Work out the finished part from the listing and answer in its coordinate system (mm). A direction names the side the tool comes from. Round coordinates to 2 decimals unless told otherwise and drop trailing zeros. Order: outer loops, then holes, each group sorted by start corner. A loop starts at its lowest first (then second) coordinate and runs counter-clockwise, first axis right, second up. Notation, with made-up numbers: M 15.5,-15 L 68.5,-15 A27 ccw 68.5,14 Z; hole C 74.5,-18 d9. An arc over 180 degrees is marked long. Return JSON: item names as keys, results as strings.
from build123d import *

# Parameters (mm, degrees)
F0_R     = 44.45
F1_DEPTH = 165.1
F2_R     = 38.1
F3_DEPTH = 254
F4_W     = 86.713158
F4_H     = 16.258716
F5_DEPTH = 25.4
F6_W     = 50.8
F6_H     = 16.258716
F7_DEPTH = 25.4
F8_R     = 2.54
F9_DEPTH = 25.4


with BuildPart() as f1:
    # F0 (on Front) → F1 (new body)
    with BuildSketch(Plane.XZ):
        Circle(F0_R)
    extrude(amount=F1_DEPTH)

    # F2 (on face) → F3 (cut)
    with BuildSketch(Plane.XZ.offset(165.1)):
        Circle(F2_R)
    extrude(amount=-F3_DEPTH, mode=Mode.SUBTRACT)

    # F4 (on Front) → F5 (join)
    with BuildSketch(Plane.XZ):
        Rectangle(F4_W, F4_H)
    extrude(amount=F5_DEPTH)

    # F6 (on face) → F7 (cut)
    with BuildSketch(Plane(origin=(0, 0, 0), x_dir=(-1, 0, 0), z_dir=(0, 1, 0))):
        Rectangle(F6_W, F6_H)
    extrude(amount=-F7_DEPTH, mode=Mode.SUBTRACT)

    # F8 (on face) → F9 (join)
    with BuildSketch(Plane.XZ.offset(25.4)):
        with Locations((31.311311, 0)):
            Circle(F8_R)
        with Locations((-31.311311, 0)):
            Circle(F8_R)
    extrude(amount=F9_DEPTH)


solid = f1.part
Item 1: Find section A-A (z = 0). Determine the outline of the cut face in (x, y), plus the area to 3 significant figures.
Output:
{"outline": "M -44.45,-165.1 L -38.1,-165.1 L -38.1,-25.4 L -33.85,-25.4 L -33.85,-50.8 L -28.77,-50.8 L -28.77,-25.4 L -25.4,-25.4 L -25.4,0 L -44.45,0 Z; M 25.4,-25.4 L 28.77,-25.4 L 28.77,-50.8 L 33.85,-50.8 L 33.85,-25.4 L 38.1,-25.4 L 38.1,-165.1 L 44.45,-165.1 L 44.45,0 L 25.4,0 Z", "area": "3,000 mm^2"}
Item 2: Find section B-B (x = 0). Determine the outline of the cut face in (y, z), plus the area to 3 significant figures.
Output:
{"outline": "M -165.1,-44.45 L 0,-44.45 L 0,-38.1 L -165.1,-38.1 Z; M -165.1,38.1 L 0,38.1 L 0,44.45 L -165.1,44.45 Z", "area": "2,100 mm^2"}
Item 3: Which of the six approach directions +Z, -Z, +X, -X, +Y, -Y give full straight-line access (tool end or side, diameter ignored) to faces 1 (the flat face through (33, -165.1, 20)), 2 (the cylindrical face through (28.774, -37.922, 0.112)), 3 (the flat face through (-31, -13, -8.129))?
Output:
{"face 1": "+Z, -Z, +X, -X, -Y", "face 2": "-Y", "face 3": "+Y, -Y"}
Item 4: Each of these flat-tipped pins is pushed along its axis until it touches: pin 1 (8 mm diameter, centred on y = -128, z = 24, fed in from +X); pin 2 (6 mm diameter, centred on x = 33, y = -15.5, fed in from -Z); pin 3 (4 mm diameter, centred on x = 9, y = -121.5, fed in from +Z). Where does it stop, or does it pass through?
Output:
{"pin 1": "stops at x = 39.7", "pin 2": "stops at z = -32.8", "pin 3": "stops at z = 43.9"}
Item 5: Find section C-C (y = -132). Determine the outline of the cut face in (x, z).
Output:
{"outline": "C 0,0 d88.9; hole C 0,0 d76.2"}
Item 6: Find section D-D (z = 21.5). Determine the outline of the cut face in (x, y), plus the area to 3 significant figures.
Output:
{"outline": "M -38.9,-165.1 L -31.45,-165.1 L -31.45,0 L -38.9,0 Z; M 31.45,-165.1 L 38.9,-165.1 L 38.9,0 L 31.45,0 Z", "area": "2,460 mm^2"}
Item 7: The mould has two halves that part along X. Classify faces 4 (the cylindrical face through (36.34, -83.71, 11.44)), 5 (the cylindrical face through (42.397, -81.394, 13.352)), 6 (the flat face through (26, 0, 0)): pulls with the +X half, pulls with the -X half, needs draft (parallel to the pull), parting line crosses it, or undercut.
Output:
{"face 4": "undercut", "face 5": "parting line crosses it", "face 6": "needs draft"}
Item 8: Consider line 1 along Z through (x, y) = (0, -41); line 2 along X through (y, z) = (-30, -1); line 3 along Y through (x, z) = (-33, -1). Determine where each line is inside the solid, lowest interval first. Write a range as [from, to].
Output:
{"line 1": "z = [-44.45, -38.1], [38.1, 44.45]", "line 2": "x = [-44.44, -38.09], [-33.65, -28.98], [28.98, 33.65], [38.09, 44.44]", "line 3": "y = [-50.8, 0]"}
